Design review of the part built by this model. Coordinates are the model's own, in mm. Give positions to 0.01 mm unless a question says otherwise; leave off trailing zeros. Write each loop counter-clockwise with the first axis right and the second up, starting at its lowest first coordinate (ties: lowest second). Pieces come first, ordered by that corner, then holes. Notation, with made-up numbers: M -13.5,13 L 4.5,13 A10 cw 4.5,26 Z; hole C 82,6 d2. An arc over 180 degrees is marked long. Write each question's results on one line, items separated by ' | '. Start each with the question number.
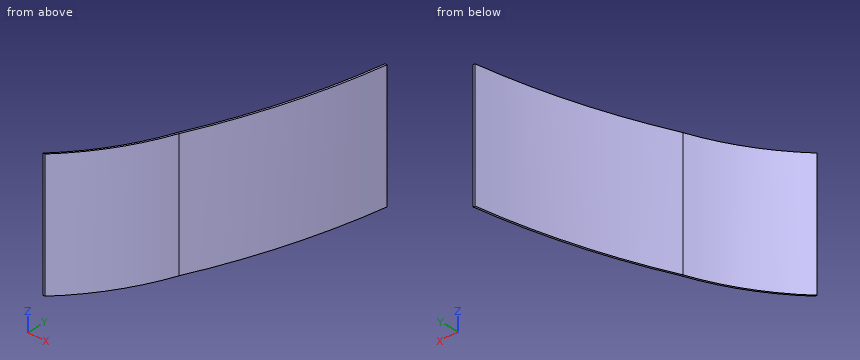
Autodesk Inventor part; units mm, degrees
ref_plane "YZ Plane" through (0, 0, 0) normal (1, 0, 0) x (0, 1, 0)
ref_plane "XZ Plane" through (0, 0, 0) normal (0, 1, 0) x (-1, 0, 0)
ref_plane "XY Plane" through (0, 0, 0) normal (0, 0, 1) x (1, 0, 0)
sketch "Sketch1" plane through (0, 0, 0) normal (0, 0, 1) x (1, 0, 0)
  arc A0 (-16.5719, 1.6749) -> (27.0317, 73.4838) centre (-157.4047, 136.334) ccw
  arc A1 (27.0317, 73.4838) -> (66.2957, 215.9257) centre (-466.9704, 286.2877) ccw
  line L0 (-16.5719, 1.6749) -> (-18.1594, 1.6749)
  line L1 (66.2957, 215.9257) -> (64.7082, 215.9257)
  arc A2 (25.4442, 73.4838) -> (64.7082, 215.9257) centre (-468.558, 286.2877) ccw
  arc A3 (-18.1594, 1.6749) -> (25.4442, 73.4838) centre (-158.9922, 136.334) ccw
  dimension "d0" = 1.5875
  dimension "d2" = 1.5875
  dimension "d3" = 537.8882
  dimension "d4" = 194.851
extrude "Extrusion1" add sketch "Sketch1" against normal blind 101.6
properties part number "Bottom Lexan Ramp" material "Polycarbonate, Clear"
Q1. For pin 1 Ø6 at (y, z) = (145.5, -31) entering from -X; pin 2 Ø3 at (x, z) = (18, -79.5) entering from -Y; pin 3 Ø2 at (x, z) = (-3.5, -23) entering from +Y, all flat-tipped, find the tip position at first contact; note any pin that passes through.
Q2. We need section C-C on y = 195. Write out the cut boundary in (x, z).
Q3. We need section A-A on z = -9. Write out the cut boundary in (x, y).
Q4. We need section B-B on x = 9.5. Write out the cut boundary in (y, z), and give its area (3 significant figures).
Q5. Wall thickness on line 1 along X through (y, z) = (78, -6); line 2 along X through (y, z) = (12, -77); line 3 along Y through (x, z) = (15.5, -93): over which ranges is each line inside the solid? List them lowest first. Write a range as from..to.
Answer sheet:
1) pin 1: x = 49.76 | pin 2: y = 48.45 | pin 3: y = 20.24
2) outline: M 61.53,-101.6 L 63.11,-101.6 L 63.11,0 L 61.53,0 Z
3) outline: M -18.16,1.67 L -16.57,1.67 A194.85 ccw 27.03,73.48 A537.89 ccw 66.3,215.93 L 64.71,215.93 A537.89 cw 25.44,73.48 A194.85 cw Z
4) outline: M 35.79,-101.6 L 38.47,-101.6 L 38.47,0 L 35.79,0 Z | area: 273 mm^2
5) line 1: 27.37..28.95 | line 2: -8.97..-7.38 | line 3: 46.5..49.62
